from build123d import *

# Parameters (mm, degrees)
SKETCH1_W                                   = 114.3
SKETCH1_H                                   = 38.1
BOSS_EXTRUDE1_DEPTH                         = 12.7
CBORE_FOR_M4_CHEESE_HEAD_SCREW2_D           = 4.5
CBORE_FOR_M4_CHEESE_HEAD_SCREW2_DEPTH       = 43.18
CBORE_FOR_M4_CHEESE_HEAD_SCREW2_CBORE_D     = 8
CBORE_FOR_M4_CHEESE_HEAD_SCREW2_CBORE_DEPTH = 2.6
CBORE_FOR_M4_CHEESE_HEAD_SCREW2_TIP         = 1.351936393
F_11_32_0_34375_DIAMETER_HOLE1_D            = 8.73125
F_11_32_0_34375_DIAMETER_HOLE1_ON_FACE_2_D  = 8.73125


with BuildPart() as part:
    # Sketch1 → Boss-Extrude1 (new body)
    with BuildSketch(Plane.XY):
        with Locations((57.15, 19.05)):
            Rectangle(SKETCH1_W, SKETCH1_H)
    extrude(amount=BOSS_EXTRUDE1_DEPTH)

    # CBORE for M4 Cheese Head Screw2
    with Locations(Plane(origin=(26.478537206, 28.204773482, 12.7), x_dir=(1, 0, 0), z_dir=(0, 0, 1))):
        with Locations((0, 0), (21.558092234, 0), (36.468605638, 0), (57.867021711, 0), (57.867021711, -19.901433884), (36.468605638, -19.901433884), (21.558092234, -19.901433884), (0, -19.901433884)):
            CounterBoreHole(CBORE_FOR_M4_CHEESE_HEAD_SCREW2_D / 2, CBORE_FOR_M4_CHEESE_HEAD_SCREW2_CBORE_D / 2, CBORE_FOR_M4_CHEESE_HEAD_SCREW2_CBORE_DEPTH, depth=CBORE_FOR_M4_CHEESE_HEAD_SCREW2_DEPTH)
            with Locations((0, 0, -(CBORE_FOR_M4_CHEESE_HEAD_SCREW2_DEPTH + CBORE_FOR_M4_CHEESE_HEAD_SCREW2_TIP / 2))):  # 118° drill point
                Cone(0, CBORE_FOR_M4_CHEESE_HEAD_SCREW2_D / 2, CBORE_FOR_M4_CHEESE_HEAD_SCREW2_TIP, mode=Mode.SUBTRACT)

    # 11/32 (0.34375) Diameter Hole1 (through all)
    with Locations(Plane(origin=(6.35, 19.05, 12.7), x_dir=(1, 0, 0), z_dir=(0, 0, 1))):
        with Locations((0, 0), (101.6, 0)):
            Hole(F_11_32_0_34375_DIAMETER_HOLE1_D / 2)

    # 11/32 (0.34375) Diameter Hole1 on face 2 (through all)
    with Locations(Plane(origin=(46.203135817, 61.386657337, 0), x_dir=(1, 0, 0), z_dir=(0, 0, 1))):
        with Locations((0, 0)):
            Hole(F_11_32_0_34375_DIAMETER_HOLE1_ON_FACE_2_D / 2)


solid = part.part
Part model, mm, in its own coordinate system. A direction names the side the tool comes from. Coordinates: 2 decimals unless noted, no trailing zeros. Order: outer loops, then holes, each group sorted by start corner. A loop starts at its lowest first (then second) coordinate and runs counter-clockwise, first axis right, second up. Notation, with made-up numbers: (12.5, 4) - (46.5, 4) arc R29 ccw to (46.5, 36) - close; hole circle Ø8 at (-13, 1.5). An arc over 180 degrees is marked (long way). Use CSV: the item, a comma, the result in double quotes.
Item 1: Mould opens along X. For faces 1 (the face through (28.726, 8.402, 4.979)), 2 (the face through (56, 38.1, 6)), 3 (the face through (114.3, 19, 6)) say: +X half, -X half, draft (parallel to the pull), parting line (faces both ways), or undercut.
Solved:
face 1,"undercut"
face 2,"draft"
face 3,"+X half"
Item 2: Saw through at C-C on z = 8.25. Give the number of separate pieces and of enclosed holes in the cut face, and give its area (3 significant figures).
Solved:
separate pieces,"1"
enclosed holes,"10"
area,"4,110 mm²"
Item 3: Saw through at B-B on y = 19.05. Give the cut face in (x, z), and give its area (3 significant figures).
Solved:
outline,"(0, 0) - (1.98, 0) - (1.98, 12.7) - (0, 12.7) - close; (10.72, 0) - (103.58, 0) - (103.58, 12.7) - (10.72, 12.7) - close; (112.32, 0) - (114.3, 0) - (114.3, 12.7) - (112.32, 12.7) - close"
area,"1,230 mm²"
Item 4: Probe probe 1 along X at (y, z) = (8, 9); probe 2 along Y at (x, z) = (49, 9); probe 3 along Y at (x, z) = (61, 10.5). List the from-to ranges inside material, lowest first.
Solved:
probe 1,"x = 0 to 24.25, 28.71 to 45.81, 50.27 to 60.72, 65.18 to 82.12, 86.58 to 114.3"
probe 2,"y = 0 to 6.27, 10.34 to 26.17, 30.24 to 38.1"
probe 3,"y = 0 to 4.81, 11.8 to 24.71, 31.7 to 38.1"
Item 5: 3-axis set-ups, long thin cutter, end or side, ignore diameter. For faces 4 (the face through (86.1, 6.6, 10.1)), 5 (the face through (82.2, 8.98, 4.98)): which of +Z, -Z, +X, -X, +Y, -Y reach the whole face in a straight line?
Solved:
face 4,"+Z"
face 5,"+Z, -Z"
Item 6: Drop flat-ended pins along their axis: P1, Ø5, axis at x = 62.95, y = 8.3, coming from the +Z side; P2, Ø2.5, axis at x = 62.95, y = 8.3, coming from the -Z side. Give the stop position or say it passes through.
Solved:
P1,"stops at z = 10.1"
P2,"passes through"
Item 7: Saw through at A-A on x = 6.35. Give the cut face in (y, z), and give its area (3 significant figures).
Solved:
outline,"(0, 0) - (14.68, 0) - (14.68, 12.7) - (0, 12.7) - close; (23.42, 0) - (38.1, 0) - (38.1, 12.7) - (23.42, 12.7) - close"
area,"373 mm²"
